Input: part model. Units: mm. Frame: model coordinates. Give positions to 0.01 mm unless a question says otherwise; leave off trailing zeros. Order: outer loops, then holes, each group sorted by start corner. A loop starts at its lowest first (then second) coordinate and runs counter-clockwise, first axis right, second up. Notation, with made-up numbers: M 16,81 L 54,81 A22 ccw 54,119 Z; hole C -14.75,53.5 d6. An arc over 180 degrees is marked long. Use a Markdown table: item, result.
Autodesk Inventor part; units mm, degrees
ref_plane "YZ Plane" through (0, 0, 0) normal (1, 0, 0) x (0, 1, 0)
ref_plane "XZ Plane" through (0, 0, 0) normal (0, 1, 0) x (-1, 0, 0)
ref_plane "XY Plane" through (0, 0, 0) normal (0, 0, 1) x (1, 0, 0)
sketch "Sketch1" plane through (0, 0, 0) normal (1, 0, 0) x (0, 1, 0)
  line L0 (0, 0) -> (0, -60)
  line L1 (0, -60) -> (6.35, -60)
  line L2 (6.35, -60) -> (6.35, 0)
  line L3 (6.35, 0) -> (0, 0)
  dimension "d0" = 60
  dimension "d1" = 6.35
extrude "Extrusion1" add sketch "Sketch1" along normal blind 6.35
sketch "Sketch2" plane through (0, 6.35, 0) normal (0, 1, 0) x (1, 0, 0)
  line L0 (0, 60) -> (0, 0)
  line L1 (0, 0) -> (4.3687, 4.3687)
  line L2 (0, 0) -> (6.1782, 0) construction
  line L3 (4.3687, 4.3687) -> (6.35, 6.35)
  line L4 (6.35, 60) -> (6.35, 0)
  line L5 (6.35, 6.35) -> (6.35, 0)
  line L6 (0, 0) -> (6.35, 0)
  line L7 (6.35, 0) -> (0, 0)
  dimension "d4" = 45
extrude "Extrusion2" cut sketch "Sketch2" against normal blind 10
sketch "Sketch3" plane through (0, 6.35, -60) normal (0, 1, 0) x (1, 0, 0)
  line L0 (0, 0) -> (6.35, -6.35)
  line L1 (6.35, 0) -> (6.35, -53.65)
  line L2 (0, 0) -> (8.9803, 0) construction
  line L3 (6.35, -6.35) -> (6.35, 0)
  line L4 (6.35, 0) -> (0, 0)
  point P0 (0, -60)
  dimension "d7" = 45
extrude "Extrusion3" cut sketch "Sketch3" against normal blind 10
properties part number "Angles in little squares"
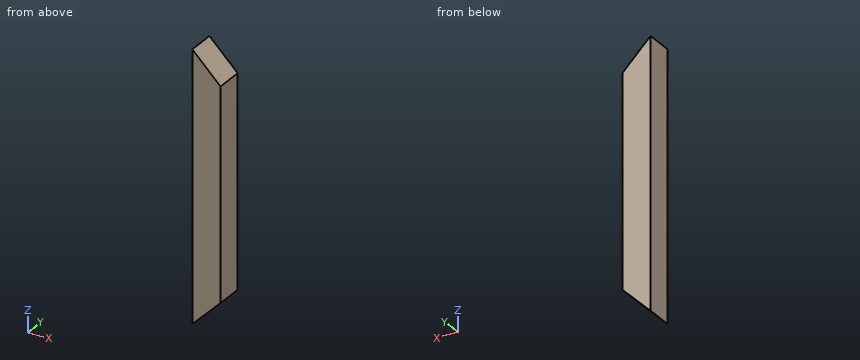
1) Material intervals for line 1 (Z direction, x = 2.5, y = 1.75); line 2 (Z direction, x = 4.5, y = 4.5); line 3 (X direction, y = 2.5, z = -6), sorted ascending. Write a range as from..to.
Response values:
| item | result |
|---|---|
| line 1 | z = -57.5..-2.5 |
| line 2 | z = -55.5..-4.5 |
| line 3 | x = 0..6 |
2) Cut plane B-B on y = 4.25. Return loops of the section in (x, z).
Response values:
| item | result |
|---|---|
| outline | M 0,-60 L 6.35,-53.65 L 6.35,-6.35 L 0,0 Z |
3) First-contact query: pin 1 Ø3 at (x, y) = (3.5, 2) entering from -Z. Flat tip, straight axial feed; report the tip coordinate or a pass-through.
Response values:
| item | result |
|---|---|
| pin 1 | stops at z = -58 |
4) Cut plane A-A on x = 4.5. Return loops of the section in (y, z).
Response values:
| item | result |
|---|---|
| outline | M 0,-55.5 L 6.35,-55.5 L 6.35,-4.5 L 0,-4.5 Z |
